Model file for the job. Use its own axes, mm. Give positions to 0.01 mm unless a question says otherwise; leave off trailing zeros. Order: outer loops, then holes, each group sorted by start corner. A loop starts at its lowest first (then second) coordinate and runs counter-clockwise, first axis right, second up. Notation, with made-up numbers: (70, 59) - (84, 59) arc R13 cw to (84, 74) - close; hole circle Ø8 at (-37, 57.5). An arc over 180 degrees is marked (long way). Use CSV: the item, a comma, the result in double quotes. Start each with the question number.
(1) Band-saw the part on A-A, the plane z = 10.45. Give the cut face in (x, y), then the cut area to 3 significant figures.
(2) Band-saw the part on B-B, the plane x = -97.25. Give the cut face in (y, z).
(3) Probe L1, parallel to X at y = -20.25, z = 10.15; L2, parallel to X at y = -22.5, z = 10.6; L3, parallel to Y at x = -98, z = 9.7. List the from-to ranges inside material, lowest first.
(4) Band-saw the part on C-C, the plane y = -21. Give the cut face in (x, z).
from build123d import *

# Parameters (mm, degrees)
CYLINDER004_R     = 5
CYLINDER004_DEPTH = 4


with BuildPart() as f_623zz:
    # Cylinder004 → Cylinder004 (new body)
    with BuildSketch(Plane(origin=(95, 22, 8), x_dir=(1, 0, 0), z_dir=(0, 0, 1))):
        Circle(CYLINDER004_R)
    extrude(amount=CYLINDER004_DEPTH)


with BuildPart() as part_mirroring011:
    # Part__Mirroring011: instance of 623ZZ
    add(f_623zz.part.mirror(Plane(origin=(0, 0, 0), x_dir=(1, 0, 0), z_dir=(0, 1, 0))))


with BuildPart() as part_mirroring015:
    # Part__Mirroring015: instance of Part__Mirroring011
    add(part_mirroring011.part.mirror(Plane(origin=(0, 0, 0), x_dir=(0, -1, 0), z_dir=(1, 0, 0))))


solid = part_mirroring015.part
Answer block:
1,outline,"circle Ø10 at (-95, -22)"
1,area,"78.5 mm2"
2,outline,"(-26.47, 8) - (-17.53, 8) - (-17.53, 12) - (-26.47, 12) - close"
3,L1,"x = -99.68 to -90.32"
3,L2,"x = -99.97 to -90.03"
3,L3,"y = -26 to -18"
4,outline,"(-99.9, 8) - (-90.1, 8) - (-90.1, 12) - (-99.9, 12) - close"
